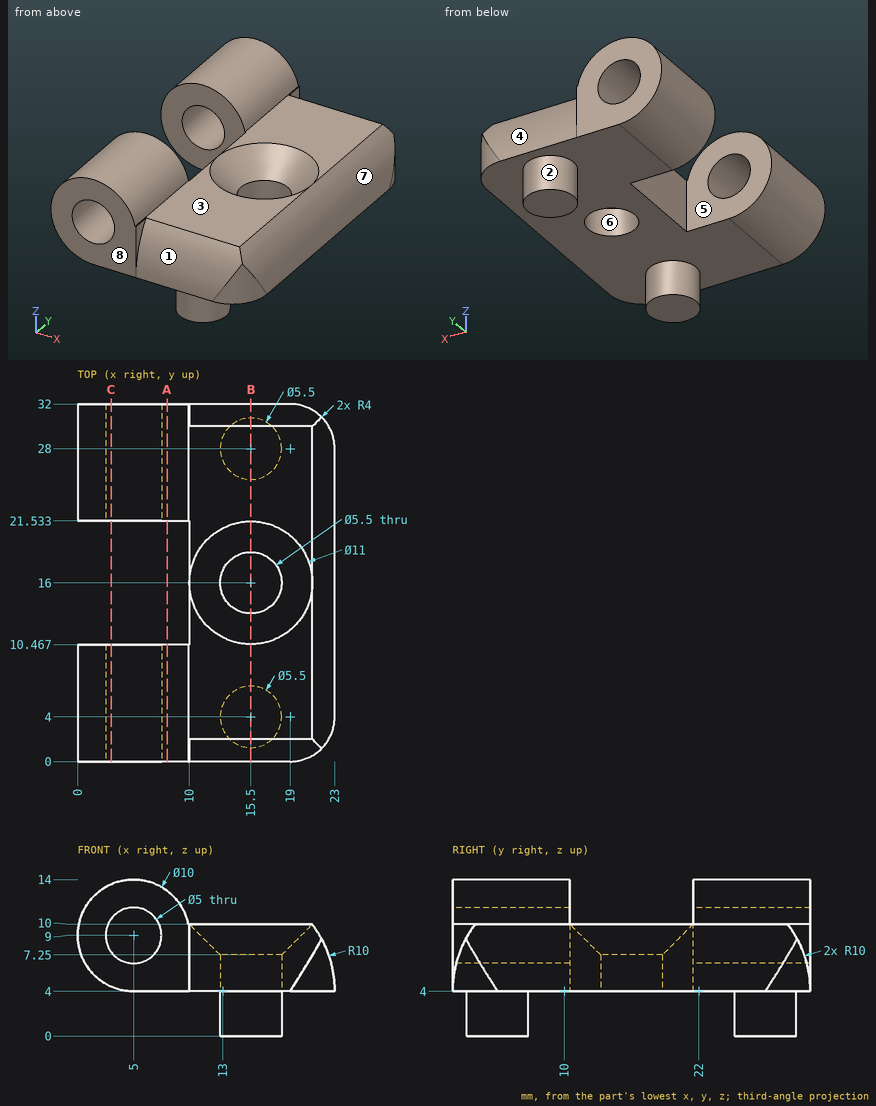
Geometry check sheet. Reference: drawing and pictorial views, mm from the part's lowest x, y, z. A direction names the side the tool comes from. Coordinates: 2 decimals unless noted, no trailing zeros. Order: outer loops, then holes, each group sorted by start corner. A loop starts at its lowest first (then second) coordinate and runs counter-clockwise, first axis right, second up.
Item 1: Scan lines: line 1 along Y through (x, z) = (8.5, 7.25); line 2 along Z through (x, y) = (5, 27.25); line 3 along Z through (x, y) = (13, 9). Record each from-to range of solid material in increasing order.
Item 2: Depth check by flat-ended pin: pin 1 (1.6 mm diameter, centred on y = 0.5, z = 8, fed in from +X); pin 2 (5.5 mm diameter, centred on x = 13.5, y = 25, fed in from +Z); pin 3 (1.5 mm diameter, centred on x = 19.5, y = 20, fed in from -Z); pin 4 (6 mm diameter, centred on x = 11.5, z = 7, fed in from -Y). Enter the tip coordinate at first touch or a pass-through.
Item 3: Section check B-B (x = 15.5). Enter the section's corners in (y, z), plus the area to 3 significant figures.
Item 4: Section check A-A (x = 8). Enter the section's corners in (y, z).
Item 5: Section check C-C (x = 3). Enter the section's corners in (y, z), plus the area to 3 significant figures.
Item 6: Tool access check on the marked faces 1, 2, 3 and 4. Record the directions out of +Z, -Z, +X, -X, +Y, -Y that give a thin tool (end or side, any length) a straight path to the whole face; none if there is none.
Item 7: Mould release check, pull along Y, two halves, no side actions. Record for the marked faces 5, 6, 7 and 8: released by +Y, released by -Y, zero draft, split by the parting line, or undercut.
Check sheet entries:
1. line 1: y = 0 to 10.47, 21.53 to 32
1. line 2: z = 4 to 6.5, 11.5 to 14
1. line 3: z = 4 to 10
2. pin 1: stops at x = 21.95
2. pin 2: stops at z = 10
2. pin 3: stops at z = 4
2. pin 4: stops at y = 0
3. outline: (0, 4) - (1.25, 4) - (1.25, 0) - (6.75, 0) - (6.75, 4) - (13.25, 4) - (13.25, 7.25) - (10.5, 10) - (2, 10) arc R10 ccw to start; (18.75, 4) - (25.25, 4) - (25.25, 0) - (30.75, 0) - (30.75, 4) - (32, 4) arc R10 ccw to (30, 10) - (21.5, 10) - (18.75, 7.25) - close
3. area: 188 mm2
4. outline: (0, 4) - (10.47, 4) - (10.47, 13) - (0, 13) - close; (21.53, 4) - (32, 4) - (32, 13) - (21.53, 13) - close
5. outline: (0, 4.42) - (10.47, 4.42) - (10.47, 7.5) - (0, 7.5) - close; (0, 10.5) - (10.47, 10.5) - (10.47, 13.58) - (0, 13.58) - close; (21.53, 4.42) - (32, 4.42) - (32, 7.5) - (21.53, 7.5) - close; (21.53, 10.5) - (32, 10.5) - (32, 13.58) - (21.53, 13.58) - close
5. area: 129 mm2
6. face 1: +Z, +X, -Y
6. face 2: -Z
6. face 3: +Z, +X, +Y, -Y
6. face 4: +Z, +X, +Y
7. face 5: undercut
7. face 6: undercut
7. face 7: zero draft
7. face 8: released by -Y
